Drawing for the job (mm, zero at the part's lowest x, y, z). A direction names the side the tool comes from. Round coordinates to 2 decimals unless told otherwise and drop trailing zeros. Write each loop counter-clockwise with the first axis right and the second up, starting at its lowest first coordinate (ties: lowest second). Pieces come first, ordered by that corner, then holes. Notation, with made-up numbers: (50.5, 37.5) -> (96.5, 37.5) arc R20 cw to (96.5, 42.5) -> close; hole circle Ø5 at (6.25, -28). An arc over 180 degrees is marked (long way). One line per question, with ' | ' between items.
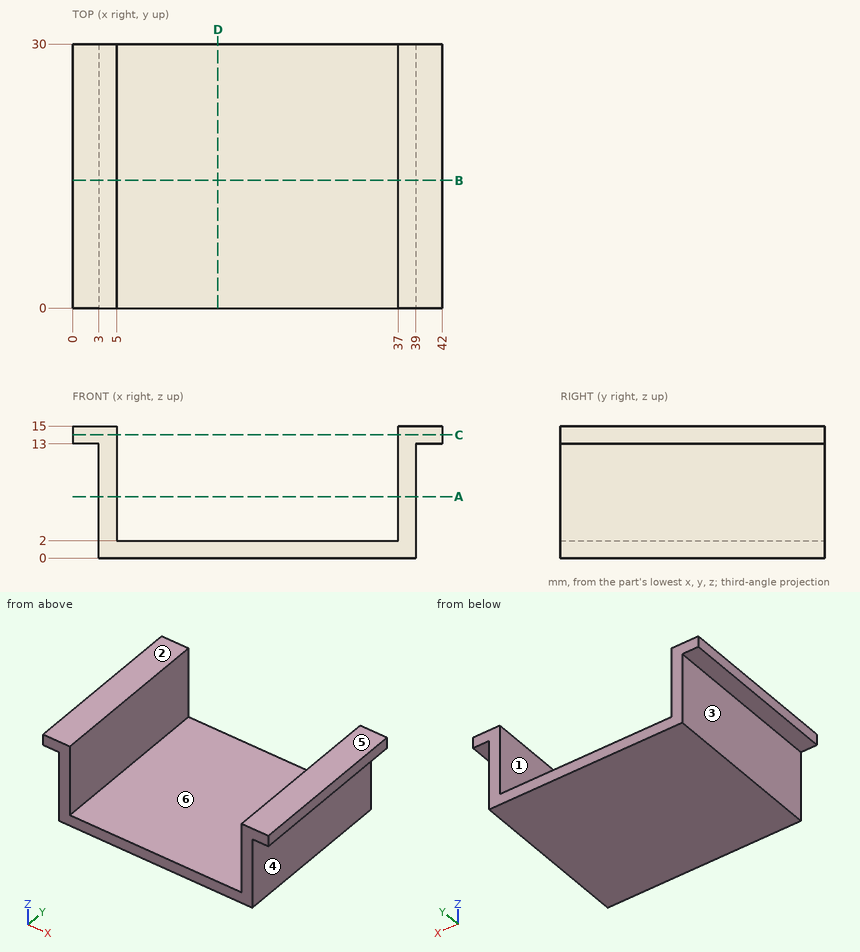
(1) Drop flat-ended pins along their axis: pin 1 (0.9 mm diameter, centred on x = 40, y = 16, fed in from -Z); pin 2 (4 mm diameter, centred on y = 7.5, z = 5.5, fed in from -X); pin 3 (4 mm diameter, centred on y = 16.5, z = 7, fed in from +X). Give the stop position or say it passes through.
Calculated:
pin 1: z = 13 | pin 2: x = 3 | pin 3: x = 39
(2) Mould opens along X. For the marked faces 4, 5 and 6 say: pulls with the +X half, pulls with the -X half, needs draft (parallel to the pull), parting line crosses it, or undercut.
Calculated:
face 4: pulls with the +X half | face 5: needs draft | face 6: undercut
(3) Slice it at B-B (y = 14.5). Write the cut outline in (x, z).
Calculated:
outline: (0, 13) -> (3, 13) -> (3, 0) -> (39, 0) -> (39, 13) -> (42, 13) -> (42, 15) -> (37, 15) -> (37, 2) -> (5, 2) -> (5, 15) -> (0, 15) -> close
(4) Slice it at A-A (z = 7). Write the cut outline in (x, y), then the cut area to 3 significant figures.
Calculated:
outline: (3, 0) -> (5, 0) -> (5, 30) -> (3, 30) -> close; (37, 0) -> (39, 0) -> (39, 30) -> (37, 30) -> close | area: 120 mm2
(5) Wall check: line 1 (X direction, y = 2, z = 5); line 2 (Z direction, x = 2, y = 6.25); line 3 (Z direction, x = 27, y = 5.75). Give the ranges that are in metal, low to high. Write a range as from..to.
Calculated:
line 1: 3..5, 37..39 | line 2: 13..15 | line 3: 0..2
(6) Slice it at C-C (z = 14). Write the cut outline in (x, y).
Calculated:
outline: (0, 0) -> (5, 0) -> (5, 30) -> (0, 30) -> close; (37, 0) -> (42, 0) -> (42, 30) -> (37, 30) -> close
(7) 3-axis set-ups, long thin cutter, end or side, ignore diameter. For the marked faces 1, 2 and 3: which of +Z, -Z, +X, -X, +Y, -Y reach the whole face in a straight line?
Calculated:
face 1: +Z, +Y, -Y | face 2: +Z, +X, -X, +Y, -Y | face 3: -Z, -X, +Y, -Y
(8) Slice it at D-D (x = 16.5). Write the cut outline in (y, z).
Calculated:
outline: (0, 0) -> (30, 0) -> (30, 2) -> (0, 2) -> close
